Geometry: final body of the model. Coordinates: model frame, mm. A direction names the side the tool comes from. Coordinates: 2 decimals unless noted, no trailing zeros. Loops run counter-clockwise (first coordinate to the right, second up) from the corner with the lowest first, then second, coordinate; pieces in that order, holes last. Notation, with made-up numbers: M -10.5,-40 L 44.5,-40 A14 cw 44.5,-33 Z; hole C 51.25,45 d1. An arc over 180 degrees is marked long. Write each question's results on one line, items separated by ' | '. Start each with the question number.
from build123d import *

# Parameters (mm, degrees)
F1_DEPTH = 22


with BuildPart() as f1:
    # F0 (on Front) → F1 (new body)
    with BuildSketch(Plane.XZ):
        with BuildLine():
            Line((460, -50), (480, -50))
            Line((480, -50), (480, 50))
            Line((480, 50), (460, 50))
            Line((460, 50), (460, 40))
            Line((460, 40), (420, 40))
            Line((420, 40), (420, 50))
            Line((420, 50), (400, 50))
            ThreePointArc((400, 50), (360.660036, 1.149579), (304.545455, 29.17011))
            ThreePointArc((304.545455, 29.17011), (300, 32.087122), (295.454545, 29.17011))
            ThreePointArc((295.454545, 29.17011), (250, 0), (204.545455, 29.17011))
            ThreePointArc((204.545455, 29.17011), (200, 32.087122), (195.454545, 29.17011))
            ThreePointArc((195.454545, 29.17011), (150, 0), (104.545455, 29.17011))
            ThreePointArc((104.545455, 29.17011), (100, 32.087122), (95.454545, 29.17011))
            ThreePointArc((95.454545, 29.17011), (50, 0), (4.545455, 29.17011))
            ThreePointArc((4.545455, 29.17011), (0, 32.087122), (-4.545455, 29.17011))
            ThreePointArc((-4.545455, 29.17011), (-50, 0), (-95.454545, 29.17011))
            ThreePointArc((-95.454545, 29.17011), (-100, 32.087122), (-104.545455, 29.17011))
            ThreePointArc((-104.545455, 29.17011), (-150, 0), (-195.454545, 29.17011))
            ThreePointArc((-195.454545, 29.17011), (-200, 32.087122), (-204.545455, 29.17011))
            ThreePointArc((-204.545455, 29.17011), (-250, 0), (-295.454545, 29.17011))
            ThreePointArc((-295.454545, 29.17011), (-300, 32.087122), (-304.545455, 29.17011))
            ThreePointArc((-304.545455, 29.17011), (-360.660036, 1.149579), (-400, 50))
            Line((-400, 50), (-420, 50))
            Line((-420, 50), (-420, 40))
            Line((-420, 40), (-460, 40))
            Line((-460, 40), (-460, 50))
            Line((-460, 50), (-480, 50))
            Line((-480, 50), (-480, -50))
            Line((-480, -50), (-460, -50))
            Line((-460, -50), (-460, -40))
            Line((-460, -40), (-420, -40))
            Line((-420, -40), (-420, -50))
            Line((-420, -50), (420, -50))
            Line((420, -50), (420, -40))
            Line((420, -40), (460, -40))
            Line((460, -40), (460, -50))
        make_face()
    extrude(amount=F1_DEPTH)


solid = f1.part
Item 1: Section C-C, the plane x = 268. Return loops of the section in (y, z).
Item 2: Section B-B, the plane x = 376.5. Return loops of the section in (y, z).
Item 3: Section A-A, the plane z = 16. Count the separate pieces of the cut face and the enclosed holes in it, plus the area to 3 significant figures.
Item 4: Contact query for flat-ended pins moving along their axis: P1, Ø11, axis at x = -442.5, y = -16, coming from the +Z side; P2, Ø8, axis at x = 316.5, y = -6.5, coming from the +Z side; P3, Ø10, axis at x = -43, y = -2.5, coming from the +Z side. Output: stop coordinate, or through.
Item 5: Set-up query: faces 1 (the flat face through (-440, -11, 40)), 2 (the flat face through (440, -11, -40)), 3 (the flat face through (-7, 0, -10)). Return all of +Z, -Z, +X, -X, +Y, -Y with unobstructed straight access to the full face (end or side cutting, diameter ignored); none if empty.
Item 6: Ray query, L1, parallel to X at y = -13, z = -41; L2, parallel to Z at x = 300, y = -16.5; L3, parallel to X at y = -15, z = 37. Return the intervals inside material, ascending. Write a range as [from, to].
Item 7: Pull-direction query (X, two-part tool) for faces 4 (the flat face through (440, -11, 40)), 5 (the flat face through (-480, -11, 1)), 6 (the cylindrical face through (-249.201, -10.846, 0.006)), 7 (the flat face through (470, -11, 50)); classes: released by +X, released by -X, zero draft, split by the parting line, or undercut.
Solutions:
1) outline: M -22,-50 L 0,-50 L 0,3.35 L -22,3.35 Z
2) outline: M -22,-50 L 0,-50 L 0,7.6 L -22,7.6 Z
3) separate pieces: 9 | enclosed holes: 0 | area: 8,220 mm²
4) P1: stops at z = 40 | P2: stops at z = 16.93 | P3: stops at z = 1.46
5) face 1: +Z, +Y, -Y | face 2: -Z, +Y, -Y | face 3: +Z, -Z, +X, -X, +Y
6) L1: x = [-480, -460], [-420, 420], [460, 480] | L2: z = [-50, 32.09] | L3: x = [-480, -398.28], [398.28, 480]
7) face 4: undercut | face 5: released by -X | face 6: undercut | face 7: zero draft
